```python
from build123d import *

# Parameters (mm, degrees)
F0_W      = 150
F0_H      = 55
F1_DEPTH  = 19
F2_R      = 17.5
F3_DEPTH  = 19.001
F4_W      = 95
F4_H      = 25
F5_DEPTH  = 19.001
F6_R      = 20
F7_R      = 10
F8_R      = 3
F9_R      = 5
F10_DEPTH = 48
F11_SIZE  = 3
F12_SIZE  = 2


with BuildPart() as f1:
    # F0 (on Front) → F1 (new body)
    with BuildSketch(Plane.XZ):
        with Locations((75, 27.5)):
            Rectangle(F0_W, F0_H)
    extrude(amount=F1_DEPTH)

    # F2 (on face) → F3 (cut, through all)
    with BuildSketch(Plane.XZ.offset(19)):
        with Locations((27.5, 27.5)):
            Circle(F2_R)
    extrude(amount=-F3_DEPTH, mode=Mode.SUBTRACT)

    # F4 (on face) → F5 (cut, through all)
    with BuildSketch(Plane.XZ.offset(19)):
        with Locations((102.5, 12.5)):
            Rectangle(F4_W, F4_H)
    extrude(amount=-F5_DEPTH, mode=Mode.SUBTRACT)

    # F6
    f6_edges = [f1.edges().sort_by_distance(p)[0] for p in [
        (55, -9.5, 25),
        (0, -9.5, 55),
    ]]
    fillet(f6_edges, radius=F6_R)

    # F7
    f7_edges = [f1.edges().sort_by_distance(p)[0] for p in [
        (150, -9.5, 25),
        (150, -9.5, 55),
    ]]
    fillet(f7_edges, radius=F7_R)

    # F8
    f8_edges = [f1.edges().sort_by_distance(p)[0] for p in [
        (107.5, -19, 25),
        (80, 0, 55),
    ]]
    fillet(f8_edges, radius=F8_R)

    # F9 (on face) → F10 (cut)
    with BuildSketch(Plane(origin=(0, 0, 0), x_dir=(1, 0, 0), z_dir=(0, 0, -1))):
        with Locations((26.9999956992, 9.4847604468)):
            Circle(F9_R)
    extrude(amount=-F10_DEPTH, mode=Mode.SUBTRACT)

    # F11
    f11_edges = [f1.edges().sort_by_distance(p)[0] for p in [
        (10, -19, 27.5),
        (10, 0, 27.5),
    ]]
    chamfer(f11_edges, length=F11_SIZE)

    # F12
    f12_edges = [f1.edges().sort_by_distance(p)[0] for p in [
        (21.999996, -9.48476, 48),
    ]]
    chamfer(f12_edges, length=F12_SIZE)


solid = f1.part
```
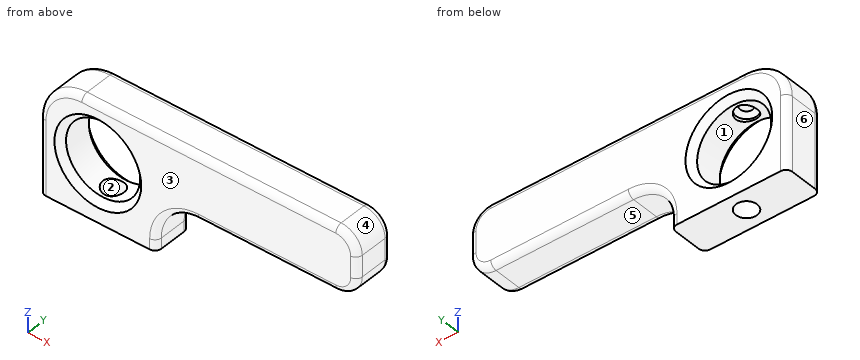
Verification items for the finished model (mm, model axes). Face numbers are marked on the shaded views. A direction names the side the tool comes from. Coordinates: 2 decimals unless noted, no trailing zeros. Write each loop counter-clockwise with the first axis right and the second up, starting at its lowest first coordinate (ties: lowest second). Pieces come first, ordered by that corner, then holes. Notation, with made-up numbers: M 51,62 L 80,62 A7 cw 80,73 Z; hole C -16,88.25 d8. An arc over 180 degrees is marked long. Answer as a JSON object with one key per item and string values. Group by question number.
(1) Release check for a two-part mould opening along X. For the marked faces 1, 2, 3 and 4 record: +X half, -X half, draft (parallel to the pull), parting line (faces both ways), or undercut.
(2) Cross-section at B-B, the plane x = 27.5. State how many separate pieces and enclosed holes the cut face has, and give its area (3 significant figures).
(3) Material ranges on line 1 (Z direction, x = 10, y = -0.75); line 2 (Z direction, x = 90, y = -10.5); line 3 (Z direction, x = 36, y = -13.75), recorded low to high.
(4) Gauge pin test, flat ends, axial feed: pin 1 (4 mm diameter, centred on x = 105.5, y = -10, fed in from -Z); pin 2 (2.5 mm diameter, centred on y = -11.5, z = 2, fed in from +X); pin 3 (1 mm diameter, centred on y = -15.5, z = 48, fed in from -X). Record the tip position at first contact, or that the pin passes through.
(5) Tool access check on the marked faces 5 and 6. Record the directions out of +Z, -Z, +X, -X, +Y, -Y that give a thin tool (end or side, any length) a straight path to the whole face; none if there is none.
(6) Cross-section at A-A, the plane y = -17.5. Record the cut outline in (x, z), and give its area (3 significant figures).
Reply:
{
 "1": {"face 1": "undercut", "face 2": "undercut", "face 3": "draft", "face 4": "+X half"},
 "2": {"separate pieces": "3", "enclosed holes": "0", "area": "233 mm²"},
 "3": {"line 1": "0 to 18.35, 36.65 to 51.14", "line 2": "25 to 55", "line 3": "0 to 12.2, 42.8 to 55"},
 "4": {"pin 1": "z = 25", "pin 2": "x = 55", "pin 3": "x = 4.39"},
 "5": {"face 5": "-Z, +X, +Y, -Y", "face 6": "+Z, -Z, -X, +Y, -Y"},
 "6": {"outline": "M 0.4,0 L 54.6,0 L 54.6,5 A20.4 cw 75,25.4 L 140,25.4 A9.6 ccw 149.6,35 L 149.6,45 A9.6 ccw 140,54.6 L 20,54.6 A19.6 ccw 0.4,35 Z; hole C 27.5,27.5 d38", "area": "4,570 mm²"}
}
